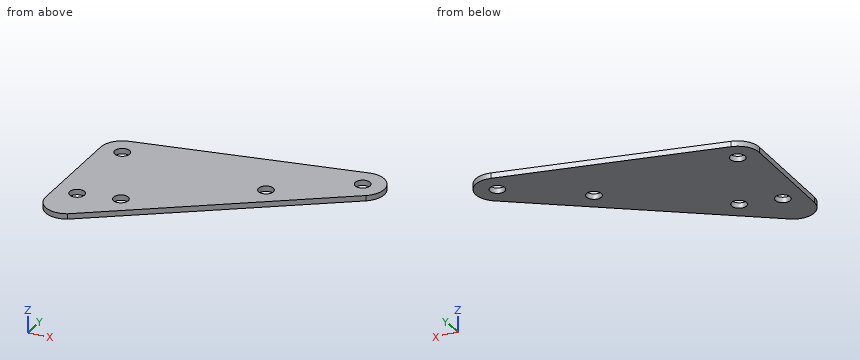
Autodesk Inventor part; units mm, degrees
ref_plane "YZ Plane" through (0, 0, 0) normal (1, 0, 0) x (0, 1, 0)
ref_plane "XZ Plane" through (0, 0, 0) normal (0, 1, 0) x (-1, 0, 0)
ref_plane "XY Plane" through (0, 0, 0) normal (0, 0, 1) x (1, 0, 0)
sketch "Sketch1" plane through (0, 0, 0) normal (0, 0, 1) x (1, 0, 0)
  ellipse E0 centre (36.5765, 33.5673) end of major axis (38.7609, 33.5673) minor radius 2.1844
  ellipse E1 centre (15.7624, 19.0472) end of major axis (13.578, 19.0472) minor radius 2.1844
  circle A0 centre (-26.9864, 20.0563) radius 2.1844
  ellipse E2 centre (-15.4587, -2.7897) end of major axis (-17.6431, -2.7897) minor radius 2.1844
  circle A1 centre (-26.9864, -5.3437) radius 2.1844
  line L0 (-33.3154, -10.8959) -> (-33.3364, 20.0563)
  arc A2 (-33.3154, -10.8959) -> (-23.9629, -16.4869) centre (-26.9654, -10.8916) ccw
  line L1 (-28.3066, 26.2675) -> (35.2563, 39.7785)
  line L2 (-23.9629, -16.4869) -> (40.2139, 28.3623)
  arc A3 (40.2139, 28.3623) -> (35.2563, 39.7785) centre (36.5765, 33.5673) ccw
  arc A4 (-28.3066, 26.2675) -> (-33.3364, 20.0563) centre (-26.9864, 20.0563) ccw
  point P0 (0, 0)
extrude "Extrusion1" add sketch "Sketch1" along normal blind 1.5875
For this review, take the finished solid that the model builds, in its own axes (mm). Coordinates: 2 decimals unless noted, no trailing zeros. Write each loop counter-clockwise with the first axis right and the second up, starting at its lowest first coordinate (ties: lowest second). Pieces come first, ordered by that corner, then holes.
(1) Add section B-B on z = 0.75. Count the separate pieces of the cut face and the enclosed holes in it, then the cut area to 3 significant figures.
(2) Add section C-C on x = 2.5. Give the boundary of the cut face in (y, z).
(3) Add section D-D on y = 24.5. Give the boundary of the cut face in (x, z), then the cut area to 3 significant figures.
(4) Add section A-A on y = -6.5. Give the boundary of the cut face in (x, z).
(5) Wall thickness on probe 1 along Y at (x, z) = (16, 0.7); probe 2 along X at (y, z) = (-3, 0.25); probe 3 along X at (y, z) = (12.5, 1.4): over which ranges is each line inside the solid? List them lowest first.
Answer sheet:
1. separate pieces: 1
1. enclosed holes: 5
1. area: 2,140 mm2
2. outline: (2.01, 0) - (32.82, 0) - (32.82, 1.59) - (2.01, 1.59) - close
3. outline: (-31.52, 0) - (34.69, 0) - (34.69, 1.59) - (-31.52, 1.59) - close
3. area: 105 mm2
4. outline: (-33.32, 0) - (-28.84, 0) - (-28.84, 1.59) - (-33.32, 1.59) - close; (-25.13, 0) - (-9.67, 0) - (-9.67, 1.59) - (-25.13, 1.59) - close
5. probe 1: y = 11.44 to 16.88, 21.22 to 35.69
5. probe 2: x = -33.32 to -17.63, -13.28 to -4.66
5. probe 3: x = -33.33 to 17.52
